Autodesk Inventor part; units mm, degrees
ref_plane "Płaszczyzna konstrukcyjna2" through (-4.3857, 4.3857, -40) normal (0, -0.7071, 0.7071) x (-1, 0, 0)
ref_plane "Płaszczyzna konstrukcyjna6" through (-4.3857, 44.3857, -40) normal (0, -0.7071, -0.7071) x (1, 0, 0)
ref_plane "Work Plane7" through (-3.0422, 31.6577, -52.7279) normal (0, 0.7071, 0.7071) x (1, 0, 0)
sketch "Szkic2" plane through (0, 0, 0) normal (0, 0, 1) x (1, 0, 0)
  circle A0 centre (0, 0) radius 2.1
  line L0 (-10, 10) -> (10, 10)
  line L1 (10, 10) -> (10, -10)
  line L2 (10, -10) -> (-10, -10)
  line L3 (-10, -10) -> (-10, 10)
  line L4 (-10, -10) -> (10, 10) construction
  line L5 (10, -10) -> (-10, 10) construction
  line L6 (-10, 8.2) -> (10, 8.2)
  line L7 (-10, -8.2) -> (10, -8.2)
  line L8 (-8.2, 10) -> (-8.2, -10)
  line L9 (10, 10) -> (30, 10)
  line L10 (30, 10) -> (30, -10)
  line L11 (30, -10) -> (10, -10)
  line L12 (10, -10) -> (10, 10)
  line L13 (-4.1857, -4.1857) -> (4.1857, -4.1857)
  line L14 (4.1857, -4.1857) -> (4.1857, 4.1857)
  line L15 (4.1857, 4.1857) -> (-4.1857, 4.1857)
  line L16 (-4.1857, 4.1857) -> (-4.1857, -4.1857)
  line L17 (-8.2, 7.1393) -> (-4.1857, 3.125)
  line L18 (-7.1393, 8.2) -> (-3.125, 4.1857)
  line L19 (-4.925, 10) -> (-3.125, 8.2)
  line L20 (4.925, 10) -> (3.125, 8.2)
  line L21 (-3.125, -8.2) -> (-4.925, -10)
  line L22 (3.125, -8.2) -> (4.925, -10)
  line L23 (-8.2, -7.1393) -> (-4.1857, -3.125)
  line L24 (-7.1393, -8.2) -> (-3.125, -4.1857)
  line L25 (3.125, -4.1857) -> (7.1393, -8.2)
  line L26 (4.1857, -3.125) -> (7.3007, -6.24)
  line L27 (4.1857, 3.125) -> (7.3007, 6.24)
  line L28 (3.125, 4.1857) -> (7.1393, 8.2)
  line L29 (-5.4993, 8.2) -> (-5.4993, 6.56)
  line L30 (5.4993, 8.2) -> (5.4993, 6.56)
  line L31 (-8.2, 5.4993) -> (-6.56, 5.4993)
  line L32 (-8.2, -5.4993) -> (-6.56, -5.4993)
  line L33 (-5.4993, -6.56) -> (-5.4993, -8.2)
  line L34 (5.4993, -6.56) -> (5.4993, -8.2)
  line L35 (-8.2, 3.125) -> (-10, 4.925)
  line L36 (-8.2, -3.125) -> (-10, -4.925)
  line L37 (7.3007, 6.24) -> (7.3007, 8.2)
  line L38 (7.3007, -6.24) -> (7.3007, -8.2)
  line L39 (15.8143, -4.1857) -> (15.8143, 4.1857)
  line L40 (24.1857, -4.1857) -> (15.8143, -4.1857)
  line L41 (23.125, -8.2) -> (24.925, -10)
  line L42 (30, -8.2) -> (10, -8.2)
  line L43 (30, 8.2) -> (10, 8.2)
  line L44 (28.2, 10) -> (28.2, -10)
  line L45 (15.8143, -3.125) -> (12.6993, -6.24)
  line L46 (27.1393, -8.2) -> (23.125, -4.1857)
  line L47 (12.6993, -6.24) -> (12.6993, -8.2)
  line L48 (16.875, -8.2) -> (15.075, -10)
  circle A1 centre (20, 0) radius 2.1
  line L49 (24.925, 10) -> (23.125, 8.2)
  line L50 (27.1393, 8.2) -> (23.125, 4.1857)
  line L51 (28.2, 7.1393) -> (24.1857, 3.125)
  line L52 (28.2, 5.4993) -> (26.56, 5.4993)
  line L53 (28.2, 3.125) -> (30, 4.925)
  line L54 (15.8143, 4.1857) -> (24.1857, 4.1857)
  line L55 (15.075, 10) -> (16.875, 8.2)
  line L56 (14.5007, 8.2) -> (14.5007, 6.56)
  line L57 (16.875, 4.1857) -> (12.8607, 8.2)
  line L58 (12.6993, 6.24) -> (12.6993, 8.2)
  line L59 (15.8143, 3.125) -> (12.6993, 6.24)
  line L60 (24.1857, 4.1857) -> (24.1857, -4.1857)
  line L61 (28.2, -7.1393) -> (24.1857, -3.125)
  line L62 (28.2, -5.4993) -> (26.56, -5.4993)
  line L63 (25.4993, -6.56) -> (25.4993, -8.2)
  line L64 (28.2, -3.125) -> (30, -4.925)
  line L65 (14.5007, -6.56) -> (14.5007, -8.2)
  line L66 (16.875, -4.1857) -> (12.8607, -8.2)
  line L67 (-13, 13) -> (33, 13)
  line L68 (33, 13) -> (33, -13)
  line L69 (33, -13) -> (-13, -13)
  line L70 (-13, -13) -> (-13, 13)
  line L71 (-10, -8.2) -> (-13, -8.2)
  line L72 (30, -8.2) -> (33, -8.2)
  line L73 (-3.125, 8.2) -> (-3.125, 10)
  line L74 (3.125, 8.2) -> (3.125, 10)
  line L75 (-8.2, 3.125) -> (-10, 3.125)
  line L76 (-8.2, -3.125) -> (-10, -3.125)
  line L77 (-3.125, -8.2) -> (-3.125, -10)
  line L78 (3.125, -8.2) -> (3.125, -10)
  line L79 (16.875, -8.2) -> (16.875, -10)
  line L80 (23.125, -8.2) -> (23.125, -10)
  line L81 (28.2, -3.125) -> (30, -3.125)
  line L82 (28.2, 3.125) -> (30, 3.125)
  line L83 (23.125, 8.2) -> (23.125, 10)
  line L84 (16.875, 8.2) -> (16.875, 10)
  line L85 (-10, 10) -> (-10, 13)
  line L86 (10, 10) -> (10, 13)
  line L87 (-5.2993, 8.2) -> (-5.2993, 6.56)
  line L88 (-6.9979, 8.3414) -> (-2.9836, 4.3271)
  line L89 (-4.3857, 4.3857) -> (4.3857, 4.3857)
  line L90 (4.3857, 4.3857) -> (4.3857, -4.3857)
  line L91 (4.3857, -4.3857) -> (-4.3857, -4.3857)
  line L92 (-4.3857, -4.3857) -> (-4.3857, 4.3857)
  line L93 (2.9836, 4.3271) -> (6.9979, 8.3414)
  line L94 (5.2993, 8.2) -> (5.2993, 6.56)
  line L95 (-10, 8) -> (10, 8)
  line L96 (10, 8) -> (30, 8)
  line L97 (2.925, 10) -> (2.925, 7.7172)
  line L98 (2.925, 7.7172) -> (5.0664, 9.8586)
  line L99 (-2.925, 10) -> (-2.925, 7.7172)
  line L100 (-2.925, 7.7172) -> (-5.0664, 9.8586)
  point P0 (0, 0)
  point P1 (0, -8.2)
  point P2 (0, 0)
  point P3 (-2.925, 8)
  point P4 (-5.2993, 8)
  point P5 (-5.2993, 6.6428)
  point P6 (-3.0422, 4.3857)
  point P7 (3.0422, 4.3857)
  point P8 (5.2993, 6.6428)
  point P9 (5.2993, 8)
  point P10 (2.925, 8)
  dimension "d2" = 4.2
  dimension "d3" = 20
  dimension "d4" = 1.8
  dimension "d5" = 20
  dimension "d6" = 20
  dimension "d7" = 1.8
  dimension "d8" = 1.8
  dimension "d9" = 1.5
  dimension "d10" = 0.75
  dimension "d11" = 135
  dimension "d12" = 6.25
  dimension "d13" = 3.125
  dimension "d14" = 1.5
  dimension "d15" = 1.5
  dimension "d16" = 1.5
  dimension "d17" = 0.75
  dimension "d18" = 0.75
  dimension "d19" = 0.75
  dimension "d20" = 1.64
  dimension "d21" = 1.64
  dimension "d22" = 1.64
  dimension "d23" = 1.64
  dimension "d24" = 1.64
  dimension "d25" = 1.64
  dimension "d26" = 45
  dimension "d27" = 1.96
  dimension "d28" = 1.96
  dimension "d29" = 3
  dimension "d30" = 3
  dimension "d31" = 3
  dimension "d32" = 3
  dimension "d49" = 0.2
  dimension "d50" = 0.2
  dimension "d51" = 0.2
  dimension "d52" = 0.2
  dimension "d53" = 0.2
  dimension "d54" = 0.2
  dimension "d55" = 0.2
  dimension "d56" = 0.2
extrude "Wyciągnięcie proste2" add sketch "Szkic2" against normal blind 40 contours L85 L67 L86 L0 | L0 L97 L6 L99 | L6 L97 L95 L99 | L100 L99 L95 L97 L98 L94 L93 L89 L88 L87 | L95 L99 L100 | L95 L98 L97
ref_plane "Płaszczyzna konstrukcyjna2" through (-4.3857, 4.3857, -40) normal (0, -0.7071, 0.7071) x (-1, 0, 0)
split "Podział1" plane through (-4.3857, 4.3857, -40) removes the side toward (0, 0.7071, -0.7071)
mirror "Odbij1" about plane through (-4.3857, 4.3857, -40) normal (0, -0.7071, 0.7071)
fillet "Zaokrąglenie1" radius 2 2 edges at (6.4625, 10, -34.3857) (-6.4625, 10, -34.3857)
sketch "Szkic7" plane through (-10, 12, -34.3857) normal (-1, 0, 0) x (0, 0, 1)
  line L0 (34.3857, -2) -> (2, -2)
  line L1 (34.3857, 1) -> (34.3857, -2)
  line L2 (34.3857, 1) -> (3, 1)
  arc A0 (0, 0) -> (2, -2) centre (2, 0) ccw
  line L3 (3, 32.3857) -> (3, 1)
  line L4 (3, 32.3857) -> (0, 32.3857)
  line L5 (0, 32.3857) -> (0, 0)
  point P0 (34.3857, -12)
extrude "Wyciągnięcie proste5" cut sketch "Szkic7" against normal blind 0.5
ref_plane "Płaszczyzna konstrukcyjna6" through (-4.3857, 44.3857, -40) normal (0, -0.7071, -0.7071) x (1, 0, 0)
split "Podział3" plane through (-4.3857, 44.3857, -40) removes the side toward (0, 0.7071, 0.7071)
sketch "Szkic8" plane through (10, 12, -34.3857) normal (1, 0, 0) x (0, 0, -1)
  line L0 (-25.7713, 1) -> (-28.7713, -2)
  line L1 (-28.7713, -2) -> (-2, -2)
  arc A0 (-2, -2) -> (0, 0) centre (-2, 0) ccw
  line L2 (0, 26.7713) -> (0, 0)
  line L3 (0, 26.7713) -> (-3, 23.7713)
  line L4 (-3, 23.7713) -> (-3, 1)
  line L5 (-25.7713, 1) -> (-3, 1)
  line L6 (-3, 23.7713) -> (-3, 1)
  line L7 (-25.7713, 1) -> (-3, 23.7713)
  point P0 (-34.3857, -12)
extrude "Wyciągnięcie proste6" add sketch "Szkic8" against normal up to surface (19.5 mm away) contours L7 L4 L5
fillet "Zaokrąglenie3" radius 2 1 edges at (0, 4.3857, -40)
ref_plane "Work Plane7" through (-3.0422, 31.6577, -52.7279) normal (0, 0.7071, 0.7071) x (1, 0, 0)
split "Split4" plane through (-3.0422, 31.6577, -52.7279) removes the side toward (0, -0.7071, -0.7071)
properties part number "Kątownik"
The model under review builds one solid part; all positions refer to its coordinate system, in mm. A direction names the side the tool comes from. Round coordinates to 2 decimals unless told otherwise and drop trailing zeros. Write each loop counter-clockwise with the first axis right and the second up, starting at its lowest first coordinate (ties: lowest second). Pieces come first, ordered by that corner, then holes. Notation, with made-up numbers: (8.25, 33) - (44.25, 33) arc R18 ccw to (44.25, 65) - close; hole circle Ø9 at (-14, 50). An arc over 180 degrees is marked (long way). One line per item, written item: value. Start each with the question number.
1. The part is to be moulded in two halves that separate along Z. For faces 6 (the face through (-9.5, 18, -26)), 7 (the face through (0.386, 24.226, -19.841)), 8 (the face through (-4, 28, -36.386)), say which applies: released by +Z, released by -Z, zero draft, split by the parting line, or undercut.
2. Machinability: for faces 1 (the face through (2.925, 9, -17)), 2 (the face through (-5.299, 29, -37)), 3 (the face through (-5.299, 7, -15)), 4 (the face through (5.299, 7, -15)), 5 (the face through (-2.925, 27, -35)), which of the approach directions +Z, -Z, +X, -X, +Y, -Y give a long, thin tool a straight path to every point of the face, cutting with its end or side? Answer none if there is none.
3. Clearance check with flat-ended pins moving along their axes: P1, Ø4, axis at x = -1, y = 26.5, coming from the +Z side; P2, Ø2, axis at x = 8, z = -21.5, coming from the -Y side; P3, Ø1, axis at y = 27.5, z = -35, coming from the +X side (3 decimals). State where each tip first meets the part, or that it passes through.
4. Consider section C-C on y = 16. Write out the cut boundary in (x, z) (3 decimals).
5. Consider section B-B on z = -9.5. Write out the cut boundary in (x, y) (3 decimals).
6. To check wall thickness, follow L1, parallel to X at y = 9, z = -12.5 (3 decimals); L2, parallel to Y at x = 5, z = -13; L3, parallel to Z at x = 5.25, y = 23.5. State the ranges of each line that lie inside material, in increasing order. Write a range as from..to.
Checks:
1. face 6: zero draft
1. face 7: released by +Z
1. face 8: undercut
2. face 1: +Z, -Z, +X
2. face 2: -Z, -X, +Y, -Y
2. face 3: +Z, -Z, -X, -Y
2. face 4: +Z, -Z, +X, -Y
2. face 5: -X, +Y, -Y
3. P1: stops at z = -20.11
3. P2: stops at y = 10
3. P3: stops at x = 2.925
4. outline: (-9.5, -34.386) - (-2.925, -34.386) - (-2.925, -36.386) - (-5.299, -36.386) - (-5.299, -37.07) - (5.299, -37.07) - (5.299, -36.386) - (2.925, -36.386) - (2.925, -34.386) - (10, -34.386) - (10, -11.614) - (-9.5, -11.614) - close
5. outline: (-9.5, 10) - (-2.925, 10) - (-2.925, 8) - (-5.299, 8) - (-5.299, 6.643) - (-3.042, 4.386) - (3.042, 4.386) - (5.299, 6.643) - (5.299, 8) - (2.925, 8) - (2.925, 10) - (10, 10) - (10, 13.886) - (-9.5, 13.886) - close
6. L1: x = -2.925..2.925
6. L2: y = 6.34..8, 10..17.39
6. L3: z = -37.79..-36.39, -34.39..-19.11
